Design review of the part built by this model. Coordinates are the model's own, in mm. Give positions to 0.01 mm unless a question says otherwise; leave off trailing zeros. Loops run counter-clockwise (first coordinate to the right, second up) from the corner with the lowest first, then second, coordinate; pieces in that order, holes last. Notation, with made-up numbers: (21.5, 18) -> (60.5, 18) arc R15 cw to (60.5, 38) -> close; hole circle Ø6 at (66, 6). An arc over 180 degrees is marked (long way). Use a Markdown table: item, result. Add a question column.
1. For pin 1 Ø6 at (x, z) = (-11.5, 3.5) entering from +Y; pin 2 Ø8 at (x, z) = (37.5, 3.5) entering from -Y; pin 3 Ø5 at (y, z) = (-10, 9) entering from +X; pin 4 Ø8 at (x, y) = (31.5, 37.5) entering from -Z, all flat-tipped, find the tip position at first contact; note any pin that passes through.
2. Add section A-A (x = 0). State the section outline as (y, z) points.
3. Add section B-B (y = -31). State the section outline as (x, z) points, and give its area (3 significant figures).
4. Add section C-C (x = -36). State the section outline as (y, z) points, and give its area (3 significant figures).
5. To check wall thickness, follow line 1 (Y direction, x = 0, z = 5.5); line 2 (Y direction, x = -4, z = 1.25); line 3 (X direction, y = -22, z = 5.5). State the ranges of each line that lie inside material, in increasing order.
6. Draft analysis for pull direction Y (two halves, no side actions). For faces 1 (the cylindrical face through (-27.963, -8.729, 0.986)), 2 (the flat face through (2, -24, 25)), 3 (the flat face through (10.691, -36.485, 0.986)), 4 (the cylindrical face through (-5.85, -26.36, 13.34)), state which applies: pulls with the +Y half, pulls with the -Y half, needs draft (parallel to the pull), parting line crosses it, or undercut.
7. Add section D-D (z = 23). State the section outline as (x, y) points.
```python
from build123d import *

# Parameters (mm, degrees)
F0_R     = 50
F0_R_2   = 27
F1_DEPTH = 2
F2_R     = 27
F2_R_2   = 23.9045
F3_DEPTH = 25


with BuildPart() as f1:
    # F0 (on Top) → F1 (new body)
    with BuildSketch(Plane.XY):
        Circle(F0_R)
        with BuildLine():
            ThreePointArc((46.986111, 0.863073), (46.992056, 0.431555), (46.994037, 0))
            ThreePointArc((46.994037, 0), (46.990732, -0.55736), (46.980816, -1.114641))
            ThreePointArc((46.980816, -1.114641), (44.654947, -14.641558), (38.519864, -26.919502))
            ThreePointArc((38.519864, -26.919502), (37.944888, -27.724087), (37.35311, -28.516394))
            ThreePointArc((37.35311, -28.516394), (27.520519, -38.092789), (15.340338, -44.419743))
            ThreePointArc((15.340338, -44.419743), (14.40225, -44.732703), (13.457784, -45.025855))
            ThreePointArc((13.457784, -45.025855), (-0.125812, -46.993869), (-13.698676, -44.953151))
            ThreePointArc((-13.698676, -44.953151), (-14.641558, -44.654947), (-15.577957, -44.336969))
            ThreePointArc((-15.577957, -44.336969), (-27.724087, -37.944888), (-37.505261, -28.315984))
            ThreePointArc((-37.505261, -28.315984), (-38.092789, -27.520519), (-38.663448, -26.712868))
            ThreePointArc((-38.663448, -26.712868), (-44.732703, -14.40225), (-46.986111, -0.863073))
            ThreePointArc((-46.986111, -0.863073), (-46.993869, 0.125812), (-46.980816, 1.114641))
            ThreePointArc((-46.980816, 1.114641), (-44.654947, 14.641558), (-38.519864, 26.919502))
            ThreePointArc((-38.519864, 26.919502), (-37.944888, 27.724087), (-37.35311, 28.516394))
            ThreePointArc((-37.35311, 28.516394), (-27.694062, 37.966807), (-15.745097, 44.277889))
            ThreePointArc((-15.745097, 44.277889), (-14.791119, 44.605631), (-13.830327, 44.912822))
            ThreePointArc((-13.830327, 44.912822), (-0.068845, 46.993987), (13.698676, 44.953151))
            ThreePointArc((13.698676, 44.953151), (14.641558, 44.654947), (15.577957, 44.336969))
            ThreePointArc((15.577957, 44.336969), (27.724087, 37.944888), (37.505261, 28.315984))
            ThreePointArc((37.505261, 28.315984), (38.092789, 27.520519), (38.663448, 26.712868))
            ThreePointArc((38.663448, 26.712868), (44.732703, 14.40225), (46.986111, 0.863073))
        make_face(mode=Mode.SUBTRACT)
        with BuildLine():
            ThreePointArc((29.29399, 0), (29.292167, 0.326733), (29.286701, 0.653426))
            ThreePointArc((29.286701, 0.653426), (27.928294, 8.840148), (24.328572, 16.317426))
            ThreePointArc((24.328572, 16.317426), (23.82963, 17.037798), (23.309365, 17.742924))
            ThreePointArc((23.309365, 17.742924), (17.398356, 23.567669), (10.091086, 27.501051))
            ThreePointArc((10.091086, 27.501051), (9.264009, 27.790573), (8.428643, 28.055228))
            ThreePointArc((8.428643, 28.055228), (0.228608, 29.293098), (-7.989748, 28.18336))
            ThreePointArc((-7.989748, 28.18336), (-8.955604, 27.891486), (-9.910836, 27.566522))
            ThreePointArc((-9.910836, 27.566522), (-17.140909, 23.755569), (-23.036737, 18.095485))
            ThreePointArc((-23.036737, 18.095485), (-23.567669, 17.398356), (-24.077513, 16.685658))
            ThreePointArc((-24.077513, 16.685658), (-27.790573, 9.264009), (-29.273371, 1.098901))
            ThreePointArc((-29.273371, 1.098901), (-29.293142, 0.222837), (-29.286701, -0.653426))
            ThreePointArc((-29.286701, -0.653426), (-27.928294, -8.840148), (-24.328572, -16.317426))
            ThreePointArc((-24.328572, -16.317426), (-23.82963, -17.037798), (-23.309365, -17.742924))
            ThreePointArc((-23.309365, -17.742924), (-17.398356, -23.567669), (-10.091086, -27.501051))
            ThreePointArc((-10.091086, -27.501051), (-9.264009, -27.790573), (-8.428643, -28.055228))
            ThreePointArc((-8.428643, -28.055228), (-0.222837, -29.293142), (8.000852, -28.180209))
            ThreePointArc((8.000852, -28.180209), (8.840148, -27.928294), (9.671534, -27.651388))
            ThreePointArc((9.671534, -27.651388), (17.037798, -23.82963), (23.036737, -18.095485))
            ThreePointArc((23.036737, -18.095485), (23.567669, -17.398356), (24.077513, -16.685658))
            ThreePointArc((24.077513, -16.685658), (27.790573, -9.264009), (29.273371, -1.098901))
            ThreePointArc((29.273371, -1.098901), (29.288834, -0.549547), (29.29399, 0))
        make_face()
        Circle(F0_R_2, mode=Mode.SUBTRACT)
        with BuildLine():
            Line((-7.989748, 28.18336), (-13.830327, 44.912822))
            ThreePointArc((-13.830327, 44.912822), (-14.791119, 44.605631), (-15.745097, 44.277889))
            Line((-15.745097, 44.277889), (-9.910836, 27.566522))
            ThreePointArc((-9.910836, 27.566522), (-8.955604, 27.891486), (-7.989748, 28.18336))
        make_face()
        with BuildLine():
            Line((-23.036737, 18.095485), (-37.35311, 28.516394))
            ThreePointArc((-37.35311, 28.516394), (-37.944888, 27.724087), (-38.519864, 26.919502))
            Line((-38.519864, 26.919502), (-24.077513, 16.685658))
            ThreePointArc((-24.077513, 16.685658), (-23.567669, 17.398356), (-23.036737, 18.095485))
        make_face()
        with BuildLine():
            Line((-29.273371, 1.098901), (-46.980816, 1.114641))
            ThreePointArc((-46.980816, 1.114641), (-46.993869, 0.125812), (-46.986111, -0.863073))
            Line((-46.986111, -0.863073), (-29.286701, -0.653426))
            ThreePointArc((-29.286701, -0.653426), (-29.293142, 0.222837), (-29.273371, 1.098901))
        make_face()
        with BuildLine():
            ThreePointArc((-38.663448, -26.712868), (-38.092789, -27.520519), (-37.505261, -28.315984))
            Line((-37.505261, -28.315984), (-23.309365, -17.742924))
            ThreePointArc((-23.309365, -17.742924), (-23.82963, -17.037798), (-24.328572, -16.317426))
            Line((-24.328572, -16.317426), (-38.663448, -26.712868))
        make_face()
        with BuildLine():
            ThreePointArc((-15.577957, -44.336969), (-14.641558, -44.654947), (-13.698676, -44.953151))
            Line((-13.698676, -44.953151), (-8.428643, -28.055228))
            ThreePointArc((-8.428643, -28.055228), (-9.264009, -27.790573), (-10.091086, -27.501051))
            Line((-10.091086, -27.501051), (-15.577957, -44.336969))
        make_face()
        with BuildLine():
            ThreePointArc((13.457784, -45.025855), (14.40225, -44.732703), (15.340338, -44.419743))
            Line((15.340338, -44.419743), (9.671534, -27.651388))
            ThreePointArc((9.671534, -27.651388), (8.840148, -27.928294), (8.000852, -28.180209))
            Line((8.000852, -28.180209), (13.457784, -45.025855))
        make_face()
        with BuildLine():
            ThreePointArc((37.35311, -28.516394), (37.944888, -27.724087), (38.519864, -26.919502))
            Line((38.519864, -26.919502), (24.077513, -16.685658))
            ThreePointArc((24.077513, -16.685658), (23.567669, -17.398356), (23.036737, -18.095485))
            Line((23.036737, -18.095485), (37.35311, -28.516394))
        make_face()
        with BuildLine():
            ThreePointArc((46.980816, -1.114641), (46.990732, -0.55736), (46.994037, 0))
            ThreePointArc((46.994037, 0), (46.992056, 0.431555), (46.986111, 0.863073))
            Line((46.986111, 0.863073), (29.286701, 0.653426))
            ThreePointArc((29.286701, 0.653426), (29.292167, 0.326733), (29.29399, 0))
            ThreePointArc((29.29399, 0), (29.288834, -0.549547), (29.273371, -1.098901))
            Line((29.273371, -1.098901), (46.980816, -1.114641))
        make_face()
        with BuildLine():
            Line((24.328572, 16.317426), (38.663448, 26.712868))
            ThreePointArc((38.663448, 26.712868), (38.092789, 27.520519), (37.505261, 28.315984))
            Line((37.505261, 28.315984), (23.309365, 17.742924))
            ThreePointArc((23.309365, 17.742924), (23.82963, 17.037798), (24.328572, 16.317426))
        make_face()
        with BuildLine():
            Line((10.091086, 27.501051), (15.577957, 44.336969))
            ThreePointArc((15.577957, 44.336969), (14.641558, 44.654947), (13.698676, 44.953151))
            Line((13.698676, 44.953151), (8.428643, 28.055228))
            ThreePointArc((8.428643, 28.055228), (9.264009, 27.790573), (10.091086, 27.501051))
        make_face()
    extrude(amount=F1_DEPTH)

    # F2 (on Top) → F3 (join)
    with BuildSketch(Plane.XY):
        Circle(F2_R)
        Circle(F2_R_2, mode=Mode.SUBTRACT)
    extrude(amount=F3_DEPTH)


solid = f1.part
```
Taken from the geometry:
| question | item | result |
|---|---|---|
| 1 | pin 1 | stops at y = 49.2 |
| 1 | pin 2 | stops at y = -36.85 |
| 1 | pin 3 | stops at x = 25.94 |
| 1 | pin 4 | stops at z = 0 |
| 2 | outline | (-50, 0) -> (-46.99, 0) -> (-46.99, 2) -> (-50, 2) -> close; (-29.29, 0) -> (-23.9, 0) -> (-23.9, 25) -> (-27, 25) -> (-27, 2) -> (-29.29, 2) -> close; (23.9, 0) -> (29.29, 0) -> (29.29, 2) -> (27, 2) -> (27, 25) -> (23.9, 25) -> close; (46.99, 0) -> (50, 0) -> (50, 2) -> (46.99, 2) -> close |
| 3 | outline | (-39.23, 0) -> (-35.32, 0) -> (-35.32, 2) -> (-39.23, 2) -> close; (-11.23, 0) -> (-9.35, 0) -> (-9.35, 2) -> (-11.23, 2) -> close; (8.91, 0) -> (10.8, 0) -> (10.8, 2) -> (8.91, 2) -> close; (35.32, 0) -> (39.23, 0) -> (39.23, 2) -> (35.32, 2) -> close |
| 3 | area | 23.2 mm^2 |
| 4 | outline | (-34.7, 0) -> (-30.21, 0) -> (-30.21, 2) -> (-34.7, 2) -> close; (-27.19, 0) -> (-24.78, 0) -> (-24.78, 2) -> (-27.19, 2) -> close; (-0.73, 0) -> (1.1, 0) -> (1.1, 2) -> (-0.73, 2) -> close; (25.13, 0) -> (27.53, 0) -> (27.53, 2) -> (25.13, 2) -> close; (30.21, 0) -> (34.7, 0) -> (34.7, 2) -> (30.21, 2) -> close |
| 4 | area | 31.3 mm^2 |
| 5 | line 1 | y = -27 to -23.9, 23.9 to 27 |
| 5 | line 2 | y = -49.84 to -46.82, -29.02 to -23.57, 23.57 to 29.02, 46.82 to 49.84 |
| 5 | line 3 | x = -15.65 to -9.35, 9.35 to 15.65 |
| 6 | face 1 | undercut |
| 6 | face 2 | needs draft |
| 6 | face 3 | undercut |
| 6 | face 4 | parting line crosses it |
| 7 | outline | circle Ø54 at (0, 0); hole circle Ø47.81 at (0, 0) |
